Could you check a few things on this model? Use its own coordinates, in mm. Face numbers are marked on the shaded views. A direction names the side the tool comes from. Round coordinates to 2 decimals unless told otherwise and drop trailing zeros. Order: outer loops, then holes, each group sorted by start corner. A loop starts at its lowest first (then second) coordinate and runs counter-clockwise, first axis right, second up. Notation, with made-up numbers: (80, 66) - (106, 66) arc R14 ccw to (106, 72) - close; hole circle Ø8 at (5, 40). An arc over 180 degrees is marked (long way). Use one line per item in the form item = value.
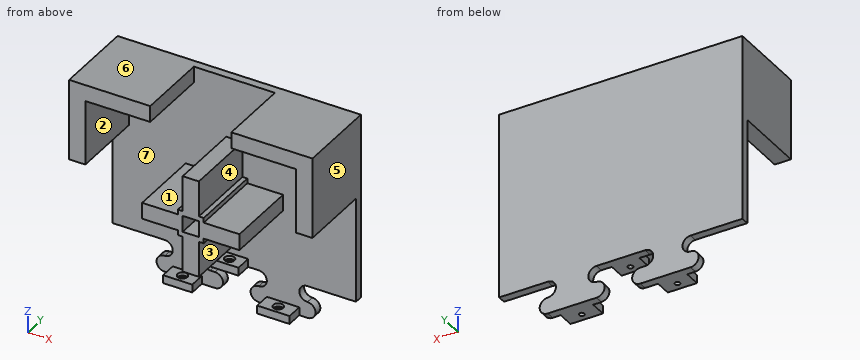
Autodesk Inventor part; units mm, degrees
ref_plane "YZ Plane" through (0, 0, 0) normal (1, 0, 0) x (0, 1, 0)
ref_plane "XZ Plane" through (0, 0, 0) normal (0, 1, 0) x (-1, 0, 0)
ref_plane "XY Plane" through (0, 0, 0) normal (0, 0, 1) x (1, 0, 0)
sketch "puzzle" plane through (0, 0, 0) normal (0, 1, 0) x (-1, 0, 0)
  line L0 (0, 0) -> (-150, 0)
  line L1 (0, -115) -> (-15, -115)
  line L2 (-135, -115) -> (-125, -115)
  line L3 (-135, -115) -> (-150, -115)
  line L4 (-75, -115) -> (-65, -115)
  line L5 (-75, -115) -> (-85.0002, -115)
  line L6 (-105, -135) -> (-94.9796, -135)
  line L7 (-94.9796, -135) -> (-115, -135)
  line L8 (-65, -115) -> (-60, -115)
  line L9 (-60, -125) -> (-63, -125)
  arc A0 (-60, -125) -> (-60, -115) centre (-60, -120) ccw
  arc A1 (-63, -125) -> (-63, -135) centre (-63, -130) ccw
  line L10 (-85.0002, -115) -> (-90.0002, -115)
  line L11 (-94.9796, -135) -> (-89.9796, -135)
  arc A2 (-90.0002, -115) -> (-90, -125) centre (-90.0002, -120) ccw
  arc A3 (-89.9796, -135) -> (-90, -125) centre (-89.9796, -130) ccw
  line L12 (-115, -135) -> (-120, -135)
  line L13 (-125, -115) -> (-120, -115)
  arc A4 (-120, -125) -> (-120, -115) centre (-120, -120) ccw
  arc A5 (-120, -125) -> (-120, -135) centre (-120, -130) ccw
  line L14 (0, -115) -> (-30, -115)
  line L15 (-63, -135) -> (-32.98, -135)
  line L16 (-32.98, -135) -> (-32, -135)
  line L17 (-30, -115) -> (-32, -115)
  arc A6 (-32, -115) -> (-32, -125) centre (-32, -120) ccw
  arc A7 (-32, -135) -> (-32, -125) centre (-32, -130) ccw
  line L18 (-150, -115) -> (-150, 0)
  line L19 (0, -115) -> (0, 0)
  dimension "d22" = 5
  dimension "d23" = 5
  dimension "d24" = 5
  dimension "d25" = 5
  dimension "d26" = 5
extrude "Extrusión1" add sketch "puzzle" along normal blind 5
sketch "peus" plane through (0, 0, 0) normal (0, -1, 0) x (1, 0, 0)
  line L0 (150, 0) -> (145, 0)
  line L1 (150, 0) -> (100, 0)
  line L2 (0, -115) -> (0, 0)
  line L3 (0, 0) -> (50, 0)
  line L4 (50, 0) -> (50, -10)
  line L5 (0, 0) -> (10, 0)
  line L6 (10, -50) -> (0, -50)
  line L7 (0, -50) -> (0, 0)
  line L8 (50, -10) -> (10, -10)
  line L9 (10, -10) -> (10, -50)
  line L10 (100, 0) -> (100, -10)
  line L11 (100, -10) -> (140, -10)
  line L12 (140, -10) -> (140, -50)
  line L13 (140, -50) -> (150, -50)
  line L14 (150, 0) -> (150, -115)
  line L15 (150, 0) -> (150, -50)
  line L16 (0, 0) -> (150, 0)
  line L17 (45, -62.5) -> (45, -72.5)
  line L18 (105, -72.5) -> (105, -62.5)
  line L19 (80, -97.5) -> (70, -97.5)
  line L20 (80, -37.5) -> (70, -37.5)
  line L21 (80, -62.5) -> (70, -62.5)
  line L22 (70, -62.5) -> (70, -72.5)
  line L23 (70, -72.5) -> (80, -72.5)
  line L24 (80, -62.5) -> (80, -72.5)
  line L25 (83, -62.5) -> (83, -59.5)
  line L26 (83, -59.5) -> (80, -59.5)
  line L27 (70, -59.5) -> (67, -59.5)
  line L28 (67, -59.5) -> (67, -62.5)
  line L29 (67, -72.5) -> (67, -75.5)
  line L30 (67, -75.5) -> (70, -75.5)
  line L31 (80, -75.5) -> (83, -75.5)
  line L32 (83, -75.5) -> (83, -72.5)
  line L33 (83, -72.5) -> (105, -72.5)
  line L34 (83, -62.5) -> (105, -62.5)
  line L35 (80, -59.5) -> (80, -37.5)
  line L36 (70, -59.5) -> (70, -37.5)
  line L37 (67, -62.5) -> (45, -62.5)
  line L38 (67, -72.5) -> (45, -72.5)
  line L39 (70, -75.5) -> (70, -97.5)
  line L40 (80, -75.5) -> (80, -97.5)
  line L41 (83, -72.5) -> (105, -72.5)
  dimension "d70" = 3
extrude "Extrusión3" add sketch "peus" along normal blind 45
sketch "Boceto4" plane through (0, 0, 0) normal (0, -1, 0) x (1, 0, 0)
  line L0 (55, -135) -> (37, -135)
  line L1 (120, -135) -> (89.9796, -135)
  line L2 (115, -135) -> (95, -135)
  line L3 (90.0002, -115) -> (60, -115)
  line L4 (75.0001, -115) -> (83.5001, -115)
  line L5 (83.5001, -115) -> (66.5001, -115)
  line L6 (83.5001, -110) -> (66.5001, -110)
  line L7 (83.5001, -110) -> (83.5001, -115)
  line L8 (66.5001, -110) -> (66.5001, -115)
  line L9 (55, -130) -> (37, -130)
  line L10 (55, -130) -> (55, -135)
  line L11 (37, -130) -> (37, -135)
  line L12 (115, -130) -> (95, -130)
  line L13 (95, -130) -> (95, -135)
  line L14 (115, -130) -> (115, -135)
  point P0 (0, 0)
extrude "Extrusión4" add sketch "Boceto4" along normal blind 10
sketch "Boceto5" plane through (55, 0, -135) normal (0, 0, -1) x (-1, 0, 0)
  circle A0 centre (9, -5) radius 1.6
  circle A1 centre (-50, -5) radius 1.6
  point P0 (55, 0)
  dimension "d81" = 3.2
  dimension "d82" = 3.2
extrude "Extrusión5" cut sketch "Boceto5" against normal blind 14.25
sketch "Boceto6" plane through (95, 0, -130) normal (0, 0, 1) x (1, 0, 0)
  circle A0 centre (-49, -5) radius 1.6
  circle A1 centre (-49, -5) radius 3.05
  circle A2 centre (10, -5) radius 1.6
  circle A3 centre (10, -5) radius 3.05
  point P0 (-95, 0)
  dimension "d85" = 6.1
  dimension "d86" = 6.1
extrude "Extrusión6" cut sketch "Boceto6" against normal blind 2
sketch "Boceto7" plane through (66.5001, 0, -110) normal (0, 0, 1) x (1, 0, 0)
  line L0 (17, -10) -> (0, -10)
  line L1 (8.5, -10) -> (8.5, 0)
  line L2 (0, 0) -> (17, 0)
  circle A0 centre (8.5, -5) radius 3.05
  point P0 (-66.5001, 0)
  dimension "d89" = 6.1
extrude "Extrusión7" cut sketch "Boceto7" against normal blind 2
sketch "Boceto8" plane through (66.5001, 0, -110) normal (0, 0, 1) x (1, 0, 0)
  circle A0 centre (8.5, -5) radius 3.05
  circle A1 centre (8.5, -5) radius 1.6
  point P0 (-66.5001, 0)
  dimension "d92" = 3.2
extrude "Extrusión8" cut sketch "Boceto8" against normal blind 13 contours A1
properties part number "base auxiliar 1"
Item 1: Will these pins go through, and if not, where does the flat tip stop? P1, Ø17.5, axis at y = -22, z = -89.5, coming from the +X side; P2, Ø17.5, axis at x = 61.5, y = -31.5, coming from the -Z side; P3, Ø2.5, axis at y = -15.5, z = -60.5, coming from the +X side.
Found:
P1 = 80
P2 = -97.5
P3 = 83
Item 2: Imagine slicing it at D-D on y = -14.5. State how many separate pieces and enclosed holes the cut face has, plus the area to 3 significant figures.
Found:
separate_pieces = 3
enclosed_holes = 1
area = 2,840 mm2
Item 3: For the marked faces 1, 2, 3 and 4, which set-ups out of +Z, -Z, +X, -X, +Y, -Y let a thin tool reach every point of the face, with its end or its side?
Found:
face_1 = -X, -Y
face_2 = -Z, -Y
face_3 = +X, -Y
face_4 = +Z, -Y
Item 4: I need wall thicknesses on L1, parallel to X at y = -5, z = -133.8; L2, parallel to Y at x = 46, z = -130.8; L3, parallel to X at y = -5, z = -111. Which ranges of each line are inside material? Lowest first, please.
Found:
L1 = 37 to 44.4, 47.6 to 55, 95 to 103.4, 106.6 to 115
L2 = -10 to -8.05, -1.95 to 5
L3 = 66.5 to 71.95, 78.05 to 83.5
Item 5: Imagine slicing it at C-C on z = -44.5. Please give me the cut outline in (x, y).
Found:
outline = (0, -45) - (10, -45) - (10, 0) - (70, 0) - (70, -45) - (80, -45) - (80, 0) - (140, 0) - (140, -45) - (150, -45) - (150, 5) - (0, 5) - close
Item 6: Imagine slicing it at B-B on x = 35. Please give me the cut outline in (y, z).
Found:
outline = (-45, -10) - (0, -10) - (0, -116) - (5, -116) - (5, 0) - (-45, 0) - close; (0, -135) - (5, -135) - (5, -124) - (0, -124) - close
Item 7: If we mould it in two halves opening along Z, with no side actions, what happens to the marked faces 5, 6 and 7? For each: released by +Z, released by -Z, zero draft, split by the parting line, or undercut.
Found:
face_5 = zero draft
face_6 = released by +Z
face_7 = undercut
Item 8: Imagine slicing it at A-A on z = -120. Please give me the cut outline in (x, y), plus the area to 3 significant figures.
Found:
outline = (37, 0) - (55, 0) - (55, 5) - (37, 5) - close; (95, 0) - (115, 0) - (115, 5) - (95, 5) - close
area = 190 mm2
